```python
from build123d import *

# Parameters (mm, degrees)
SKETCH1_R           = 1.5
SKETCH1_R_2         = 4.7
BOSS_EXTRUDE1_DEPTH = 3
SKETCH2_W           = 25
SKETCH2_H           = 12
BOSS_EXTRUDE3_DEPTH = 3
SKETCH4_R           = 2
CUT_EXTRUDE2_DEPTH  = 31.33101416
BOSS_EXTRUDE4_DEPTH = 1.5


with BuildPart() as part:
    # Sketch1 → Boss-Extrude1 (new body)
    with BuildSketch(Plane(origin=(0, 0, 0), x_dir=(1, 0, 0), z_dir=(0, 1, 0))):
        with BuildLine():
            ThreePointArc((21.045480929, 12.95727721), (19.873908054, 15.785704335), (17.045480929, 16.95727721))
            Line((17.045480929, 16.95727721), (2.545480929, 16.95727721))
            ThreePointArc((2.545480929, 16.95727721), (-0.282946196, 15.785704335), (-1.454519071, 12.95727721))
            Line((-1.454519071, 12.95727721), (-1.454519071, -19.89272279))
            Line((-1.454519071, -19.89272279), (2.724413117, -19.89272279))
            Line((2.724413117, -19.89272279), (16.866548741, -19.89272279))
            Line((16.866548741, -19.89272279), (21.045480929, -19.89272279))
            Line((21.045480929, -19.89272279), (21.045480929, 12.95727721))
        make_face()
        with Locations(Location((1.045480929, -14.84272279, 0), (0, 0, 270))):
            Circle(SKETCH1_R, mode=Mode.SUBTRACT)
        with Locations(Location((18.545480929, -14.84272279, 0), (0, 0, 270))):
            Circle(SKETCH1_R, mode=Mode.SUBTRACT)
        with Locations(Location((9.795480929, 5.75727721, 0), (0, 0, 270))):
            Circle(SKETCH1_R_2, mode=Mode.SUBTRACT)
    extrude(amount=BOSS_EXTRUDE1_DEPTH)

    # Sketch2 → Boss-Extrude3 (add)
    with BuildSketch(Plane(origin=(21.045480929, 0, 0), x_dir=(0, 0, -1), z_dir=(1, 0, 0))):
        with Locations((0.45727721, -6)):
            Rectangle(SKETCH2_W, SKETCH2_H)
    extrude(amount=-BOSS_EXTRUDE3_DEPTH)

    # Sketch4 → Cut-Extrude2 (cut, through all)
    with BuildSketch(Plane.ZY.offset(-18.045480929)):
        with Locations((7.324019086, -6)):
            Circle(SKETCH4_R)
        with Locations((-7.324019086, -6)):
            Circle(SKETCH4_R)
    extrude(amount=-CUT_EXTRUDE2_DEPTH, mode=Mode.SUBTRACT)

    # Sketch5 → Boss-Extrude4 (add, symmetric)
    with BuildSketch(Plane.XY.offset(2.04272279)):
        Polygon((18.045480929, -4.641213544), (11.011197959, 0), (18.045480929, 0), align=None)
    extrude(amount=BOSS_EXTRUDE4_DEPTH, both=True)


solid = part.part
```
Source: CAD feature listing. Evaluate the final solid. Frame: model axes, mm. A direction names the side the tool comes from. Coordinates: 2 decimals unless noted, no trailing zeros. Write each loop counter-clockwise with the first axis right and the second up, starting at its lowest first coordinate (ties: lowest second). Pieces come first, ordered by that corner, then holes. Notation, with made-up numbers: (13, -37) - (17, -37) arc R21 ccw to (17, -31) - close; hole circle Ø5 at (63, -30.5). An arc over 180 degrees is marked (long way). Answer as a JSON object with one key per item and string values.
Q1. Draft query along Z for faces 6 (the cylindrical face through (19.52, -7.22, 5.74)), 7 (the cylindrical face through (19.52, -7.22, -8.91)), 8 (the flat face through (20, -12, 0)), 9 (the flat face through (15, -2, 0.543)). Return one class per face: released by +Z, released by -Z, zero draft, split by the parting line, or undercut.
Ans:
{"face 6": "undercut", "face 7": "undercut", "face 8": "zero draft", "face 9": "released by -Z"}
Q2. Section query B-B, the plane x = 5.5. Output: boundary loops of the cut face in (y, z), plus the area to 3 significant figures.
Ans:
{"outline": "(0, -16.96) - (3, -16.96) - (3, -7.66) - (0, -7.66) - close; (0, -3.85) - (3, -3.85) - (3, 19.89) - (0, 19.89) - close", "area": "99.1 mm2"}
Q3. Material intervals for line 1 (Y direction, x = 5.5, z = 0); line 2 (X direction, y = -10.25, z = 8.5); line 3 (Z direction, x = 8, y = 2), sorted ascending. Write a range as [from, to].
Ans:
{"line 1": "y = [0, 3]", "line 2": "x = [18.05, 21.05]", "line 3": "z = [-16.96, -10.1], [-1.41, 19.89]"}
Q4. Section query D-D, the plane z = 1. Output: boundary loops of the cut face in (x, y), plus the area to 3 significant figures.
Ans:
{"outline": "(-1.45, 0) - (11.01, 0) - (18.05, -4.64) - (18.05, -12) - (21.05, -12) - (21.05, 3) - (-1.45, 3) - close", "area": "120 mm2"}
Q5. Set-up query: faces 1 (the flat face through (15, -2, 3.543)), 2 (the flat face through (20, -6, 12.043)), 3 (the cylindrical face through (5.626, 1.479, -3.589)), 4 (the flat face through (18.045, -6, 0)), 5 (the flat face through (20, -6, -12.957)). Return all of +Z, -Z, +X, -X, +Y, -Y with unobstructed straight access to the full face (end or side cutting, diameter ignored); none if empty.
Ans:
{"face 1": "+Z, -X, -Y", "face 2": "+Z, +X, -X, -Y", "face 3": "+Y, -Y", "face 4": "-X, -Y", "face 5": "-Z, +X, -X, -Y"}
Q6. Section query C-C, the plane z = 7. Output: boundary loops of the cut face in (x, y), plus the area to 3 significant figures.
Ans:
{"outline": "(-1.45, 0) - (18.05, 0) - (18.05, -4.03) - (21.05, -4.03) - (21.05, 3) - (-1.45, 3) - close; (18.05, -12) - (21.05, -12) - (21.05, -7.97) - (18.05, -7.97) - close", "area": "91.7 mm2"}
Q7. First-contact query: pin 1 Ø2 at (x, y) = (18.5, -1.5) entering from -Z; pin 2 Ø1.4 at (x, y) = (13, -2) entering from +Z; pin 3 Ø3.5 at (x, y) = (14, -1) entering from -Z; pin 4 Ø7 at (x, z) = (6, -6.5) entering from -Y. Flat tips, straight axial feed; report the tip coordinate or a pass-through.
Ans:
{"pin 1": "stops at z = -12.96", "pin 2": "stops at z = 3.54", "pin 3": "stops at z = -16.96", "pin 4": "stops at y = 0"}
Q8. Section query A-A, the plane y = -6. Output: boundary loops of the cut face in (x, z).
Ans:
{"outline": "(18.05, -12.96) - (21.05, -12.96) - (21.05, -9.32) - (18.05, -9.32) - close; (18.05, -5.32) - (21.05, -5.32) - (21.05, 5.32) - (18.05, 5.32) - close; (18.05, 9.32) - (21.05, 9.32) - (21.05, 12.04) - (18.05, 12.04) - close"}
